Read the model definition and answer for the solid it produces. Units are mm, in the model's axes. Coordinates: 2 decimals unless noted, no trailing zeros. Order: outer loops, then holes, each group sorted by start corner. A loop starts at its lowest first (then second) coordinate and runs counter-clockwise, first axis right, second up. Notation, with made-up numbers: (84, 79) -> (114, 79) arc R18 ccw to (114, 89) -> close; hole circle Ø5 at (29, 85). An arc over 180 degrees is marked (long way). Answer as a JSON object with one key per item and string values. Group by question number.
1) Section B-B on y = 9.25 is taken. Determine the outline of the cut face in (x, z).
2) Section A-A on z = 0.1 is taken. Determine the outline of the cut face in (x, y), and give its area (3 significant figures).
3) Consider L1, parallel to X at y = 14.5, z = 0.05; L2, parallel to X at y = 3.75, z = 0.05; L3, parallel to Y at x = 35.5, z = -0.15. Determine where each line is inside the solid, lowest interval first.
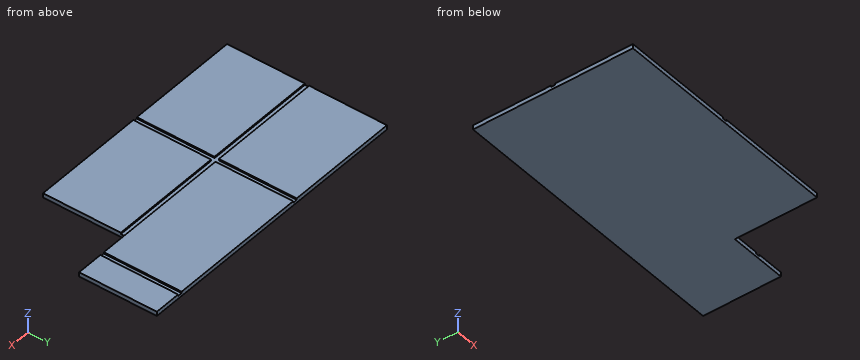
Autodesk Inventor part; units mm, degrees
ref_plane "YZ Plane" through (0, 0, 0) normal (1, 0, 0) x (0, 1, 0)
ref_plane "XZ Plane" through (0, 0, 0) normal (0, 1, 0) x (-1, 0, 0)
ref_plane "XY Plane" through (0, 0, 0) normal (0, 0, 1) x (1, 0, 0)
sketch "Sketch1" plane through (0, 0, 0) normal (0, 0, 1) x (1, 0, 0)
  line L0 (0, 0) -> (32, 0)
  line L1 (32, 0) -> (32, 22)
  line L2 (32, 22) -> (0, 22)
  line L3 (0, 22) -> (0, 0)
  line L4 (0, 11) -> (0, 10.7)
  line L5 (0, 10.7) -> (0, 11.3)
  line L6 (32, 16.3) -> (32, 15.7)
  line L7 (0, 15.7) -> (0, 11.3)
  line L8 (16.3, 22) -> (15.7, 22)
  line L9 (15.7, 22) -> (16.3, 22)
  line L10 (16.3, 0) -> (15.7, 0)
  line L11 (32, 11) -> (32, 11.3)
  line L12 (0, 11.3) -> (0, 10.7)
  line L13 (32, 10.7) -> (32, 11.3)
  line L14 (16.3, 22) -> (15.7, 22)
  line L15 (15.7, 0) -> (16.3, 0)
  line L16 (0, 10.7) -> (15.7, 10.7)
  line L17 (16.3, 10.7) -> (32, 10.7)
  line L18 (16.3, 0) -> (16.3, 10.7)
  line L19 (16.3, 11.3) -> (16.3, 22)
  line L20 (32, 11.3) -> (16.3, 11.3)
  line L21 (15.7, 11.3) -> (0, 11.3)
  line L22 (15.7, 22) -> (15.7, 11.3)
  line L23 (15.7, 10.7) -> (15.7, 0)
  line L24 (32, 11.3) -> (40, 11.3)
  line L25 (40, 11.3) -> (40, 22)
  line L26 (40, 22) -> (32, 22)
  line L27 (32, 22) -> (32, 11.3)
  line L28 (36, 22) -> (36.3, 22)
  line L29 (36.3, 22) -> (35.7, 22)
  line L30 (35.7, 22) -> (35.7, 11.3)
  line L31 (35.7, 11.3) -> (36.3, 11.3)
  line L32 (36.3, 11.3) -> (36.3, 22)
  point P0 (36.3, 16.3)
  dimension "d1" = 22
  dimension "d6" = 0.6
  dimension "d14" = 0.3
  dimension "d15" = 0.6
  dimension "d16" = 0.6
  dimension "d17" = 8
  dimension "d18" = 0.3
  dimension "d19" = 0.6
extrude "Extrusion1" add sketch "Sketch1" against normal blind 0.4
extrude "Extrusion2" add sketch "Sketch1" along normal blind 0.2 contours L3 L16 L23 L0 | L18 L17 L1 L0 | L3 L2 L22 L21 | L20 L19 L2 L1 | L1 L26 L30 L24 | L32 L26 L25 L24
properties part number "Wire Position"
Worked answers:
{
 "1": {"outline": "(0, -0.4) -> (32, -0.4) -> (32, 0.2) -> (16.3, 0.2) -> (16.3, 0) -> (15.7, 0) -> (15.7, 0.2) -> (0, 0.2) -> close"},
 "2": {"outline": "(0, 0) -> (15.7, 0) -> (15.7, 10.7) -> (0, 10.7) -> close; (0, 11.3) -> (15.7, 11.3) -> (15.7, 22) -> (0, 22) -> close; (16.3, 0) -> (32, 0) -> (32, 10.7) -> (16.3, 10.7) -> close; (16.3, 11.3) -> (35.7, 11.3) -> (35.7, 22) -> (16.3, 22) -> close; (36.3, 11.3) -> (40, 11.3) -> (40, 22) -> (36.3, 22) -> close", "area": "751 mm²"},
 "3": {"L1": "x = 0 to 15.7, 16.3 to 35.7, 36.3 to 40", "L2": "x = 0 to 15.7, 16.3 to 32", "L3": "y = 11.3 to 22"}
}
